```python
from build123d import *

# Parameters (mm, degrees)
F0_W     = 2000
F0_H     = 900
F1_DEPTH = 5
F2_W     = 10
F2_H     = 900
F3_DEPTH = 1000
F5_DEPTH = 2000.001
F7_D     = 12


with BuildPart() as f1:
    # F0 (on Front) → F1 (new body, symmetric)
    with BuildSketch(Plane.XZ):
        Rectangle(F0_W, F0_H)
    extrude(amount=F1_DEPTH, both=True)

    # F2 (on face) → F3 (join)
    with BuildSketch(Plane.XZ.offset(5)):
        with Locations((-995, 0)):
            Rectangle(F2_W, F2_H)
        with Locations((995, 0)):
            Rectangle(F2_W, F2_H)
    extrude(amount=F3_DEPTH)

    # F4 (on face) → F5 (cut, through all)
    with BuildSketch(Plane.YZ.offset(1000)):
        Polygon((-105, -450), (-1005, 450), (-1005, -450), align=None)
    extrude(amount=-F5_DEPTH, mode=Mode.SUBTRACT)

    # F7 (through all)
    with Locations(Plane(origin=(-1000, 0, 0), x_dir=(0, -1, 0), z_dir=(-1, 0, 0))):
        with Locations((345, 400), (55, -181.721583)):
            Hole(F7_D / 2)


solid = f1.part
```
Geometry check sheet. Reference: the model listing, model coordinates, mm. A direction names the side the tool comes from. Round coordinates to 2 decimals unless told otherwise and drop trailing zeros. Loops run counter-clockwise (first coordinate to the right, second up) from the corner with the lowest first, then second, coordinate; pieces in that order, holes last. Notation, with made-up numbers: (-10.5, 31.25) - (24.5, 31.25) arc R35 ccw to (24.5, 70.25) - close; hole circle Ø8 at (-1.75, 3.5). An arc over 180 degrees is marked (long way). Use a Markdown table: item, result.
Q1. Cross-section at D-D on x = 557. Record the cut outline in (y, z), plus the area to 3 significant figures.
Solutions:
| item | result |
|---|---|
| outline | (-5, -450) - (5, -450) - (5, 450) - (-5, 450) - close |
| area | 9,000 mm2 |
Q2. Material ranges on line 1 (X direction, y = -252, z = 237); line 2 (Z direction, x = -992.75, y = -55); line 3 (Y direction, x = 552, z = 252), recorded low to high.
Solutions:
| item | result |
|---|---|
| line 1 | x = -1000 to -990, 990 to 1000 |
| line 2 | z = -450 to -187.72, -175.72 to 450 |
| line 3 | y = -5 to 5 |
Q3. Cross-section at B-B on z = 109. Record the cut outline in (x, y), plus the area to 3 significant figures.
Solutions:
| item | result |
|---|---|
| outline | (-1000, -664) - (-990, -664) - (-990, -5) - (990, -5) - (990, -664) - (1000, -664) - (1000, 5) - (-1000, 5) - close |
| area | 33,200 mm2 |
Q4. Go/stop test with flat-tipped pins: P1, Ø9.5, axis at y = -345, z = 400, coming from the +X side; P2, Ø1.5, axis at x = 8.5, z = -45.5, coming from the -Y side. Record where each tip stops, or that it passes through.
Solutions:
| item | result |
|---|---|
| P1 | passes through |
| P2 | stops at y = -5 |
Q5. Cross-section at C-C on y = -378. Record the cut outline in (x, z), plus the area to 3 significant figures.
Solutions:
| item | result |
|---|---|
| outline | (-1000, -177) - (-990, -177) - (-990, 450) - (-1000, 450) - close; (990, -177) - (1000, -177) - (1000, 450) - (990, 450) - close |
| area | 12,500 mm2 |
Q6. Access from +Z, -Z, +X, -X, +Y, -Y to the whole of each face (thin tool, end or side, straight path). Record for faces 1 (the flat face through (-14, 5, 6)), 2 (the flat face through (-990, -387, 94)).
Solutions:
| item | result |
|---|---|
| face 1 | +Z, -Z, +X, -X, +Y |
| face 2 | +Z, -Z, -Y |
Q7. Cross-section at A-A on y = -862.5. Record the cut outline in (x, z), plus the area to 3 significant figures.
Solutions:
| item | result |
|---|---|
| outline | (-1000, 307.5) - (-990, 307.5) - (-990, 450) - (-1000, 450) - close; (990, 307.5) - (1000, 307.5) - (1000, 450) - (990, 450) - close |
| area | 2,850 mm2 |
